For this review, take the finished solid that the model builds, in its own axes (mm). A direction names the side the tool comes from. Coordinates: 2 decimals unless noted, no trailing zeros. Loops run counter-clockwise (first coordinate to the right, second up) from the corner with the lowest first, then second, coordinate; pieces in that order, holes last. Notation, with made-up numbers: M -15.75,85 L 3.25,85 A12 cw 3.25,93 Z; hole C 27.25,72 d6. An arc over 180 degrees is marked long. Answer as a JSON object with one key per item and string values. Group by question number.
Item 1: Wall thickness on L1, parallel to X at y = -1.25, z = -28.5; L2, parallel to Z at x = 19.5, y = 4.75; L3, parallel to X at y = -6.25, z = -26.5: over which ranges is each line inside the solid? List them lowest first. Write a range as from..to.
Item 2: Add section A-A (y = 10.5). State the section outline as (x, z) points.
Item 3: Insertion check: pin 1 (4 mm diameter, centred on y = 2, z = -30.5, fed in from -X); pin 2 (1.5 mm diameter, centred on y = 1, z = -30, fed in from +X); pin 3 (2 mm diameter, centred on x = 24.5, y = -8.5, fed in from +Z). Each pin has a flat end and moves straight along its axis. Give the tip position at first contact, or say it passes through.
Item 4: Add section C-C (z = 29). State the section outline as (x, y) points, then the cut area to 3 significant figures.
Item 5: Add section B-B (x = 9.5). State the section outline as (y, z) points.
Item 6: Tool access review of faces 1 (the face through (-30.462, -0.178, 27.182)), 2 (the face through (29, 0, -6.215)), 3 (the face through (-29, 0, -6.215)): name each direction out of +Z, -Z, +X, -X, +Y, -Y from which nothing blocks a thin tool from reaching the whole face with its end or side.
from build123d import *

# Parameters (mm, degrees)
F1_DEPTH      = 12.7
F1_DEPTH_BACK = 12.7


with BuildPart() as f1:
    # F0 (on Front) → F1 (new body, two sides)
    with BuildSketch(Plane.XZ) as f1_sk:
        with BuildLine():
            Line((12.7, 34.4253193842), (0, 34.4253193842))
            Line((0, 34.4253193842), (0, -5.8595561422))
            Line((0, -5.8595561422), (0, -6.2146806158))
            Line((0, -6.2146806158), (19.245794032, -6.2146806158))
            Line((19.245794032, -6.2146806158), (38.1, -6.2146806158))
            Line((38.1, -6.2146806158), (38.1, 9.0253193842))
            ThreePointArc((38.1, 9.0253193842), (30.6605122421, 26.9858316263), (12.7, 34.4253193842))
        make_face()
        with BuildLine():
            Line((0, -5.8595561422), (0, 34.4253193842))
            Line((0, 34.4253193842), (-12.7, 34.4253193842))
            ThreePointArc((-12.7, 34.4253193842), (-30.6605122421, 26.9858316263), (-38.1, 9.0253193842))
            Line((-38.1, 9.0253193842), (-38.1, -6.2146806158))
            Line((-38.1, -6.2146806158), (-19.245794032, -6.2146806158))
            Line((-19.245794032, -6.2146806158), (0, -5.8595561422))
        make_face()
        Polygon((0, -6.2146806158), (0, -5.8595561422), (-19.245794032, -6.2146806158), align=None)
        Polygon((19.245794032, -6.2146806158), (0, -6.2146806158), (-19.245794032, -6.2146806158), (-7.6351859607, -44.2130304873), (7.6351859607, -44.2130304873), align=None)
    extrude(amount=F1_DEPTH)
    extrude(f1_sk.sketch, amount=-F1_DEPTH_BACK)


solid = f1.part
From the geometry:
{
 "1": {"L1": "x = -12.44..12.44", "L2": "z = -6.21..33.5", "L3": "x = -13.05..13.05"},
 "2": {"outline": "M -38.1,-6.21 L -19.25,-6.21 L -7.64,-44.21 L 7.64,-44.21 L 19.25,-6.21 L 38.1,-6.21 L 38.1,9.03 A25.4 ccw 12.7,34.43 L -12.7,34.43 A25.4 ccw -38.1,9.03 Z"},
 "3": {"pin 1": "stops at x = -12.44", "pin 2": "stops at x = 12.21", "pin 3": "stops at z = 32.01"},
 "4": {"outline": "M -28.39,-12.7 L 28.39,-12.7 L 28.39,12.7 L -28.39,12.7 Z", "area": "1,440 mm²"},
 "5": {"outline": "M -12.7,-38.11 L 12.7,-38.11 L 12.7,34.43 L -12.7,34.43 Z"},
 "6": {"face 1": "+Z, -X, +Y, -Y", "face 2": "-Z, +X, +Y, -Y", "face 3": "-Z, -X, +Y, -Y"}
}
